Work out the finished part from the listing and answer in its coordinate system (mm). A direction names the side the tool comes from. Round coordinates to 2 decimals unless told otherwise and drop trailing zeros. Order: outer loops, then holes, each group sorted by start corner. A loop starts at its lowest first (then second) coordinate and runs counter-clockwise, first axis right, second up. Notation, with made-up numbers: (64, -2.5) - (82, -2.5) arc R29 cw to (82, 17.5) - close; hole circle Ø4 at (88.5, 2). An arc over 180 degrees is marked (long way). Answer in a Markdown table with one row per item.
from build123d import *

# Parameters (mm, degrees)
SKETCH1_W           = 152.4
SKETCH1_H           = 76.2
BOSS_EXTRUDE1_DEPTH = 12.7
FILLET1_R           = 2.54
SKETCH3_W           = 133.99496637
SKETCH3_H           = 57.912
CUT_EXTRUDE4_DEPTH  = 13.7
FILLET2_R           = 2.54
SKETCH2_W           = 10.16
SKETCH2_H           = 2.54
CUT_EXTRUDE5_DEPTH  = 12.7
SKETCH4_R           = 2.794
CUT_EXTRUDE6_DEPTH  = 12.7
SKETCH5_R           = 2.794
CUT_EXTRUDE7_DEPTH  = 12.7


with BuildPart() as part:
    # Sketch1 → Boss-Extrude1 (new body)
    with BuildSketch(Plane(origin=(0, 0, 0), x_dir=(1, 0, 0), z_dir=(0, 1, 0))):
        Rectangle(SKETCH1_W, SKETCH1_H)
    extrude(amount=BOSS_EXTRUDE1_DEPTH)

    # Fillet1
    fillet1_edges = [part.edges().sort_by_distance(p)[0] for p in [
        (76.2, 6.35, 38.1),
        (-76.2, 6.35, 38.1),
        (-76.2, 6.35, -38.1),
        (76.2, 6.35, -38.1),
    ]]
    fillet(fillet1_edges, radius=FILLET1_R)

    # Sketch3 → Cut-Extrude4 (cut, through all)
    with BuildSketch(Plane(origin=(0, 0, 0), x_dir=(1, 0, 0), z_dir=(0, 1, 0))):
        Rectangle(SKETCH3_W, SKETCH3_H)
    extrude(amount=CUT_EXTRUDE4_DEPTH, mode=Mode.SUBTRACT)

    # Fillet2
    fillet2_edges = [part.edges().sort_by_distance(p)[0] for p in [
        (66.997483185, 6.35, 28.956),
        (66.997483185, 6.35, -28.956),
        (-66.997483185, 6.35, -28.956),
        (-66.997483185, 6.35, 28.956),
    ]]
    fillet(fillet2_edges, radius=FILLET2_R)

    # Sketch2 → Cut-Extrude5 (cut)
    with BuildSketch(Plane.ZY.offset(76.2)):
        with Locations((-20.32, 11.43)):
            Rectangle(SKETCH2_W, SKETCH2_H)
    extrude(amount=-CUT_EXTRUDE5_DEPTH, mode=Mode.SUBTRACT)

    # Sketch4 → Cut-Extrude6 (cut)
    with BuildSketch(Plane(origin=(0, 0, 0), x_dir=(1, 0, 0), z_dir=(0, 1, 0))):
        with Locations((-70.612, 32.512)):
            Circle(SKETCH4_R)
    extrude(amount=CUT_EXTRUDE6_DEPTH, mode=Mode.SUBTRACT)

    # Sketch5 → Cut-Extrude7 (cut)
    with BuildSketch(Plane(origin=(0, 0, 0), x_dir=(1, 0, 0), z_dir=(0, 1, 0))):
        with Locations((70.612, -32.512)):
            Circle(SKETCH5_R)
    extrude(amount=CUT_EXTRUDE7_DEPTH, mode=Mode.SUBTRACT)


solid = part.part
1) This flat-tipped pin is pushed along its axis until it touches: pin 1 (3 mm diameter, centred on x = -73, z = -22.5, fed in from +Y). Where does it stop, or does it pass through?
Filled in:
| item | result |
|---|---|
| pin 1 | stops at y = 10.16 |
2) Find section C-C, the plane y = 2.75. Give the vertices of the cut face in (x, z).
Filled in:
| item | result |
|---|---|
| outline | (-76.2, -35.56) arc R2.54 ccw to (-73.66, -38.1) - (73.66, -38.1) arc R2.54 ccw to (76.2, -35.56) - (76.2, 35.56) arc R2.54 ccw to (73.66, 38.1) - (-73.66, 38.1) arc R2.54 ccw to (-76.2, 35.56) - close; hole circle Ø5.59 at (-70.61, -32.51); hole (-67, -26.42) arc R2.54 ccw to (-64.46, -28.96) - (64.46, -28.96) arc R2.54 ccw to (67, -26.42) - (67, 26.42) arc R2.54 ccw to (64.46, 28.96) - (-64.46, 28.96) arc R2.54 ccw to (-67, 26.42) - close; hole circle Ø5.59 at (70.61, 32.51) |
3) Find section A-A, the plane z = 5. Give the vertices of the cut face in (x, y).
Filled in:
| item | result |
|---|---|
| outline | (-76.2, 0) - (-67, 0) - (-67, 12.7) - (-76.2, 12.7) - close; (67, 0) - (76.2, 0) - (76.2, 12.7) - (67, 12.7) - close |
4) Find the intervals of material crossed by probe 1 along X at (y, z) = (2, -15); probe 2 along Z at (x, y) = (-34, 7.5); probe 3 along X at (y, z) = (11.5, -18.5), in increasing order. Write a range as from..to.
Filled in:
| item | result |
|---|---|
| probe 1 | x = -76.2..-67, 67..76.2 |
| probe 2 | z = -38.1..-28.96, 28.96..38.1 |
| probe 3 | x = 67..76.2 |
5) Which of the six approach directions +Z, -Z, +X, -X, +Y, -Y give full straight-line access (tool end or side, diameter ignored) to faces 1 (the face through (76.2, 6, 0)), 2 (the face through (-72, 10.16, -20)), 3 (the face through (-66.997, 6, 0))?
Filled in:
| item | result |
|---|---|
| face 1 | +Z, -Z, +X, +Y, -Y |
| face 2 | -X, +Y |
| face 3 | +Y, -Y |
6) The mould has two halves that part along Z. Classify faces 4 (the face through (68.553, 6.261, 30.624)), 5 (the face through (-1, 6, -38.1)), 6 (the face through (11, 12.7, 31)), 7 (the face through (-1, 6, 38.1)): released by +Z, released by -Z, zero draft, split by the parting line, or undercut.
Filled in:
| item | result |
|---|---|
| face 4 | undercut |
| face 5 | released by -Z |
| face 6 | zero draft |
| face 7 | released by +Z |
7) Find section B-B, the plane x = -30.5. Give the vertices of the cut face in (y, z), then the cut area to 3 significant figures.
Filled in:
| item | result |
|---|---|
| outline | (0, -38.1) - (12.7, -38.1) - (12.7, -28.96) - (0, -28.96) - close; (0, 28.96) - (12.7, 28.96) - (12.7, 38.1) - (0, 38.1) - close |
| area | 232 mm^2 |
